Autodesk Inventor part; units mm, degrees
ref_plane "YZ Plane" through (0, 0, 0) normal (1, 0, 0) x (0, 1, 0)
ref_plane "XZ Plane" through (0, 0, 0) normal (0, 1, 0) x (-1, 0, 0)
ref_plane "XY Plane" through (0, 0, 0) normal (0, 0, 1) x (1, 0, 0)
sketch "Sketch1" plane through (0, 0, 0) normal (0, 0, 1) x (1, 0, 0)
  line L0 (-12.1708, 16.0073) -> (13.2292, 16.0073)
  line L1 (13.2292, 16.0073) -> (13.2292, -34.7927)
  line L2 (13.2292, -34.7927) -> (-12.1708, -34.7927)
  line L3 (-12.1708, -34.7927) -> (-12.1708, 16.0073)
  line L4 (11.9592, 14.7373) -> (-10.9008, 14.7373)
  line L5 (-10.9008, 14.7373) -> (-10.9008, -33.5227)
  line L6 (-10.9008, -33.5227) -> (11.9592, -33.5227)
  line L7 (11.9592, -33.5227) -> (11.9592, 14.7373)
  point P0 (0, 0)
  dimension "d0" = 25.4
  dimension "d1" = 50.8
  dimension "d2" = 1.27
extrude "Extrusion1" add sketch "Sketch1" along normal blind 203.2
sketch "Sketch2" plane through (-12.1708, 16.0073, 0) normal (0, 1, 0) x (1, 0, 0)
  circle A0 centre (12.7, -12.7) radius 1.7272
  line L0 (25.4, 0) -> (0, 0)
  line L1 (0, 0) -> (0, -203.2)
  point P0 (12.1708, 0)
  dimension "d5" = 3.4544
  dimension "d6" = 12.7
  dimension "d7" = 12.7
extrude "Extrusion2" cut sketch "Sketch2" against normal through all
pattern_linear "Rectangular Pattern1" count 20 spacing 25.4 along (0, 0, 1) of "Extrusion2"
sketch "Sketch4" plane through (13.2292, -34.7927, 0) normal (1, 0, 0) x (0, 0, -1)
  circle A0 centre (-159.639, 25.4) radius 14.2875
  line L0 (0, 0) -> (0, 50.8)
  line L1 (0, 50.8) -> (-203.2, 50.8)
  point P0 (0, 34.7927)
  dimension "d41" = 28.575
  dimension "d42" = 159.639
  dimension "d43" = 25.4
extrude "Extrusion4" cut sketch "Sketch4" against normal through all
equation "\"d3\" = d13"
equation "\"d10\" = d14"
equation "\"d13\" = 203.2"
equation "\"d14\" = d13"
equation "\"d32\" = 101.6"
properties part number "VersaFrame 28in"
Geometry: final body of the model. Coordinates: model frame, mm. A direction names the side the tool comes from. Coordinates: 2 decimals unless noted, no trailing zeros. Order: outer loops, then holes, each group sorted by start corner. A loop starts at its lowest first (then second) coordinate and runs counter-clockwise, first axis right, second up.
(1) Access query for faces 1 (the face through (0.3, 15.38, 112.59)), 2 (the face through (11.959, -10, 100)). Directions: +Z, -Z, +X, -X, +Y, -Y. A direction counts if a zero-diameter tool reaches every point of the face in a straight line with its end or side. Return the directions, or none.
(2) Section query C-C (z = 190.5). Return the cut outline in (x, y).
(3) Section query A-A (x = -9). Return the cut outline in (y, z).
(4) Section query B-B (y = -29). Return the cut outline in (x, z), plus the area to 3 significant figures.
(5) Section query D-D (y = -2). Return the cut outline in (x, z).
(6) Draft query along X for faces 3 (the face through (0, -33.523, 100)), 4 (the face through (-12.171, -10, 100)), 5 (the face through (1, -34.793, 100)). Return one class per face: pulls with the +X half, pulls with the -X half, needs draft (parallel to the pull), parting line crosses it, or undercut.
(7) Material intervals for probe 1 along X at (y, z) = (7.5, 96); probe 2 along Y at (x, z) = (-7, 39.5); probe 3 along X at (y, z) = (-34.4, 190.5), sorted ascending.
Solution:
1. face 1: +Y, -Y
1. face 2: +Z, -Z
2. outline: (-12.17, -34.79) - (-1.2, -34.79) - (-1.2, -33.52) - (-10.9, -33.52) - (-10.9, 14.74) - (-1.2, 14.74) - (-1.2, 16.01) - (-12.17, 16.01) - close; (2.26, -34.79) - (13.23, -34.79) - (13.23, 16.01) - (2.26, 16.01) - (2.26, 14.74) - (11.96, 14.74) - (11.96, -33.52) - (2.26, -33.52) - close
3. outline: (-34.79, 0) - (-33.52, 0) - (-33.52, 203.2) - (-34.79, 203.2) - close; (14.74, 0) - (16.01, 0) - (16.01, 203.2) - (14.74, 203.2) - close
4. outline: (-12.17, 0) - (-10.9, 0) - (-10.9, 203.2) - (-12.17, 203.2) - close; (11.96, 0) - (13.23, 0) - (13.23, 203.2) - (11.96, 203.2) - close
4. area: 516 mm2
5. outline: (-12.17, 0) - (-10.9, 0) - (-10.9, 147.41) - (-12.17, 147.41) - close; (-12.17, 171.87) - (-10.9, 171.87) - (-10.9, 203.2) - (-12.17, 203.2) - close; (11.96, 0) - (13.23, 0) - (13.23, 147.41) - (11.96, 147.41) - close; (11.96, 171.87) - (13.23, 171.87) - (13.23, 203.2) - (11.96, 203.2) - close
6. face 3: undercut
6. face 4: pulls with the -X half
6. face 5: needs draft
7. probe 1: x = -12.17 to -10.9, 11.96 to 13.23
7. probe 2: y = -34.79 to -33.52, 14.74 to 16.01
7. probe 3: x = -12.17 to -1.2, 2.26 to 13.23
